Input: part model. Units: mm. Frame: model coordinates. A direction names the side the tool comes from. Coordinates: 2 decimals unless noted, no trailing zeros. Write each loop counter-clockwise with the first axis right and the second up, starting at its lowest first coordinate (ties: lowest second). Pieces come first, ordered by that corner, then holes. Notation, with made-up numbers: (9, -34) - (36, -34) arc R32 cw to (36, -5) - close; hole circle Ø10 at (-33.75, 79). An arc over 180 degrees is marked (long way). One line per question, with ' | ' between items. Start each with the question number.
1) Section query C-C on x = -1.25. Return loops of the section in (y, z).
2) Line query: line 1 (X direction, y = 0.15, z = -1.05); line 2 (Y direction, x = -9, z = -0.6); line 3 (Y direction, x = -8.5, z = -0.3). Output: solid intervals per line, ascending.
3) First-contact query: P1, Ø1.5, axis at x = -1.5, y = -1, coming from the -Z side; P2, Ø1, axis at x = -9, z = 0, coming from the -Y side; P3, Ø1, axis at x = -9.5, y = 1, coming from the +Z side. Flat tips, straight axial feed; report the tip coordinate or a pass-through.
4) Section query D-D on x = -5.75. Return loops of the section in (y, z).
5) Section query A-A on z = 0. Return loops of the section in (x, y).
6) Reachability of faces 1 (the cylindrical face through (-1, 0, -1)), 2 (the flat face through (0, 0, 0)), 3 (the cylindrical face through (-9, 0, -1)) from +Z, -Z, +X, -X, +Y, -Y: full face, straight path, thin tool, end or side. Return the list, or none.
Autodesk Inventor part; units mm, degrees
ref_plane "YZ Plane" through (0, 0, 0) normal (1, 0, 0) x (0, 1, 0)
ref_plane "XZ Plane" through (0, 0, 0) normal (0, 1, 0) x (-1, 0, 0)
ref_plane "XY Plane" through (0, 0, 0) normal (0, 0, 1) x (1, 0, 0)
sketch "Boceto1" plane through (0, 0, 0) normal (0, 0, 1) x (1, 0, 0)
  line L0 (0, 0) -> (-11, 0)
  line L1 (0, 0) -> (-11, 0)
  line L2 (-11, 0) -> (-11, 1)
  line L3 (0, 1) -> (0, 0)
  line L4 (-8, 0) -> (-2, 0)
  line L5 (-2, 0) -> (-2, 1.5)
  line L6 (-2, 1.5) -> (-8, 1.5)
  line L7 (-8, 1.5) -> (-8, 0)
  line L8 (-11, 1) -> (-8, 1)
  line L9 (-2, 1) -> (0, 1)
  dimension "d1" = 2
  dimension "d2" = 2
  dimension "d3" = 3
  dimension "d4" = 3
  dimension "d5" = 2
  dimension "d6" = 6
  dimension "d7" = 11
revolve "Revolución1" add sketch "Boceto1" angle 360 about axis through (0, 0, 0) along (-1, 0, 0)
thread "Rosca1"
thread "Rosca2"
properties part number "Hudson 1-64"
Answer key:
1) outline: circle Ø2 at (0, 0)
2) line 1: -8 to -2 | line 2: -0.8 to 0.8 | line 3: -0.95 to 0.95
3) P1: z = -1.43 | P2: y = -1 | P3: z = 0.87
4) outline: circle Ø3 at (0, 0)
5) outline: (-11, -1) - (-8, -1) - (-8, -1.5) - (-2, -1.5) - (-2, -1) - (0, -1) - (0, 1) - (-2, 1) - (-2, 1.5) - (-8, 1.5) - (-8, 1) - (-11, 1) - close
6) face 1: +X | face 2: +Z, -Z, +X, +Y, -Y | face 3: -X
